Design review of the part built by this model. Coordinates are the model's own, in mm. Give positions to 0.01 mm unless a question says otherwise; leave off trailing zeros. Write each loop counter-clockwise with the first axis right and the second up, starting at its lowest first coordinate (ties: lowest second). Pieces come first, ordered by that corner, then holes. Notation, with made-up numbers: (58, 63) -> (99, 63) arc R27 ccw to (99, 91) -> close; hole circle Ø2 at (51, -33). An arc over 180 degrees is marked (long way). Answer as a JSON object with one key per item and string values.
Autodesk Inventor part; units mm, degrees
ref_plane "YZ Plane" through (0, 0, 0) normal (1, 0, 0) x (0, 1, 0)
ref_plane "XZ Plane" through (0, 0, 0) normal (0, 1, 0) x (-1, 0, 0)
ref_plane "XY Plane" through (0, 0, 0) normal (0, 0, 1) x (1, 0, 0)
sketch "Sketch1" plane through (0, 0, 0) normal (0, 0, 1) x (1, 0, 0)
  arc A0 (-10.8675, 2) -> (-10.8675, -2) centre (0, 0) ccw
  line L0 (16, -2) -> (-16, -2)
  line L1 (-16, -2) -> (-16, 2)
  line L2 (-16, 2) -> (16, 2)
  line L3 (16, 2) -> (16, -2)
  line L4 (16, -2) -> (-16, 2) construction
  line L5 (-16, -2) -> (16, 2) construction
  arc A1 (10.8675, 2) -> (-10.8675, 2) centre (0, 0) ccw
  arc A2 (-10.8675, -2) -> (10.8675, -2) centre (0, 0) ccw
  line L6 (30, -15) -> (-30, -15)
  line L7 (-30, -15) -> (-30, 15)
  line L8 (-30, 15) -> (30, 15)
  line L9 (30, 15) -> (30, -15)
  line L10 (30, -15) -> (-30, 15) construction
  line L11 (-30, -15) -> (30, 15) construction
  arc A3 (10.8675, -2) -> (10.8675, 2) centre (0, 0) ccw
  dimension "d0" = 22.1
  dimension "d1" = 32
  dimension "d2" = 4
  dimension "d3" = 60
  dimension "d4" = 30
extrude "Extrusion1" add sketch "Sketch1" along normal blind 2
fillet "Fillet1" radius 2 4 edges at (30, 15, 1) (-30, 15, 1) (30, -15, 1) (-30, -15, 1)
properties part number "HeatSink-sheet-H2mm"
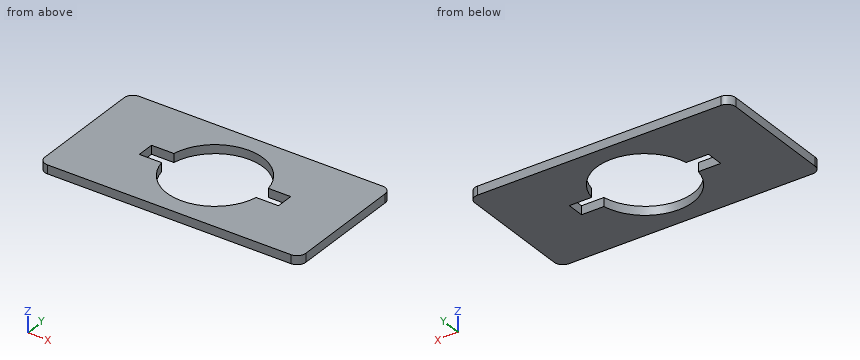
(1) We need section B-B, the plane z = 0.85. State the section outline as (x, y) points, then the cut area to 3 significant figures.
Here are the results:
{"outline": "(-30, -13) arc R2 ccw to (-28, -15) -> (28, -15) arc R2 ccw to (30, -13) -> (30, 13) arc R2 ccw to (28, 15) -> (-28, 15) arc R2 ccw to (-30, 13) -> close; hole (-16, -2) -> (-10.87, -2) arc R11.05 ccw to (10.87, -2) -> (16, -2) -> (16, 2) -> (10.87, 2) arc R11.05 ccw to (-10.87, 2) -> (-16, 2) -> close", "area": "1,370 mm²"}
(2) For line 1 along X through (y, z) = (1.75, 1.1); line 2 along Y through (x, z) = (-13, 1.75); line 3 along X through (y, z) = (-9, 1.4), list the stretches that pass through material, from the lowest coordinate up.
Here are the results:
{"line 1": "x = -30 to -16, 16 to 30", "line 2": "y = -15 to -2, 2 to 15", "line 3": "x = -30 to -6.41, 6.41 to 30"}
(3) We need section A-A, the plane y = 9.75. State the section outline as (x, z) points.
Here are the results:
{"outline": "(-30, 0) -> (-5.2, 0) -> (-5.2, 2) -> (-30, 2) -> close; (5.2, 0) -> (30, 0) -> (30, 2) -> (5.2, 2) -> close"}
(4) We need section C-C, the plane x = -7.5. State the section outline as (y, z) points.
Here are the results:
{"outline": "(-15, 0) -> (-8.11, 0) -> (-8.11, 2) -> (-15, 2) -> close; (8.11, 0) -> (15, 0) -> (15, 2) -> (8.11, 2) -> close"}
